```python
from build123d import *

# Parameters (mm, degrees)
SKETCH1_R                 = 2.85
SKETCH1_R_2               = 2
BOSS_EXTRUDE1_DEPTH       = 60
SKETCH1_4_R               = 2
BOSS_EXTRUDE2_DEPTH       = 7
M4X0_7_TAPPED_HOLE1_D     = 3.3
M4X0_7_TAPPED_HOLE1_DEPTH = 10.1
M4X0_7_TAPPED_HOLE1_TIP   = 0.991420021
CHAMFER1_SIZE             = 0.5


with BuildPart() as part:
    # Sketch1 → Boss-Extrude1 (new body)
    with BuildSketch(Plane(origin=(0, 0, 0), x_dir=(1, 0, 0), z_dir=(0, 1, 0))):
        with Locations(Location((0, 0, 0), (0, 0, 270))):
            Circle(SKETCH1_R)
        Circle(SKETCH1_R_2, mode=Mode.SUBTRACT)
        Circle(SKETCH1_R_2)
    extrude(amount=BOSS_EXTRUDE1_DEPTH)

    # Sketch1_4 → Boss-Extrude2 (add)
    with BuildSketch(Plane(origin=(0, 0, 0), x_dir=(1, 0, 0), z_dir=(0, 1, 0))):
        with Locations(Location((0, 0, 0), (0, 0, 270))):
            Circle(SKETCH1_4_R)
    extrude(amount=-BOSS_EXTRUDE2_DEPTH)

    # M4x0.7 Tapped Hole1
    with Locations(Plane(origin=(0, 60, 0), x_dir=(1, 0, 0), z_dir=(0, 1, 0))):
        with Locations((0, 0)):
            Hole(M4X0_7_TAPPED_HOLE1_D / 2, depth=M4X0_7_TAPPED_HOLE1_DEPTH)
            with Locations((0, 0, -(M4X0_7_TAPPED_HOLE1_DEPTH + M4X0_7_TAPPED_HOLE1_TIP / 2))):  # 118° drill point
                Cone(0, M4X0_7_TAPPED_HOLE1_D / 2, M4X0_7_TAPPED_HOLE1_TIP, mode=Mode.SUBTRACT)

    # Chamfer1
    chamfer1_edges = [part.edges().sort_by_distance(p)[0] for p in [
        (0, -7, -2),
    ]]
    chamfer(chamfer1_edges, length=CHAMFER1_SIZE)


solid = part.part
```
Model file for the job. Use its own axes, mm. A direction names the side the tool comes from. Give positions to 0.01 mm unless a question says otherwise; leave off trailing zeros. Order: outer loops, then holes, each group sorted by start corner. A loop starts at its lowest first (then second) coordinate and runs counter-clockwise, first axis right, second up.
1) Wall check: probe 1 along Y at (x, z) = (-2.1, -0.65); probe 2 along Z at (x, y) = (-1.9, 39); probe 3 along Z at (x, y) = (1.55, 10.5). Give the ranges that are in metal, low to high.
2) Saw through at B-B, the plane y = 7.5. Write the cut outline in (x, z).
3) Pin check, flat tip, straight feed: pin 1 (1 mm diameter, centred on x = -1, z = -2, fed in from -Y). Stop position of the tip, or through.
4) Saw through at A-A, the plane y = 51. Write the cut outline in (x, z), then the cut area to 3 significant figures.
5) 3-axis set-ups, long thin cutter, end or side, ignore diameter. For faces 4 (the cylindrical face through (-2, -3, 0)), 5 (the flat face through (0, -7, 0)), 6 (the cylindrical face through (1.216, 54.879, -1.115)): which of +Z, -Z, +X, -X, +Y, -Y reach the whole face in a straight line?
6) Mould opens along X. For faces 1 (the conical face through (-0.1, 49.1, 0.3)), 2 (the cylindrical face through (-1.734, 29.58, -2.262)), 3 (the flat face through (-2, 60, 0)) say: +X half, -X half, draft (parallel to the pull), parting line (faces both ways), or undercut.
Computed:
1. probe 1: y = 0 to 60
1. probe 2: z = -2.12 to 2.12
1. probe 3: z = -2.39 to 2.39
2. outline: circle Ø5.7 at (0, 0)
3. pin 1: stops at y = -6.76
4. outline: circle Ø5.7 at (0, 0); hole circle Ø3.3 at (0, 0)
4. area: 17.0 mm2
5. face 4: -Y
5. face 5: +Z, -Z, +X, -X, -Y
5. face 6: +Y
6. face 1: undercut
6. face 2: parting line
6. face 3: draft
